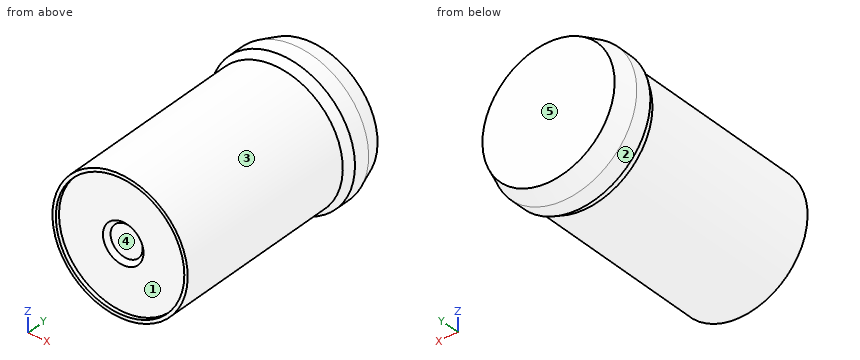
from build123d import *

# Parameters (mm, degrees)
FILLET1_SIZE = 1.5


with BuildPart() as part:
    # Sketch1 → Revolve1 (revolve)
    with BuildSketch(Plane.XY, mode=Mode.PRIVATE) as revolve1_sk:
        Polygon((20, 0), (20, 56.727116956), (21.5, 59.325193167), (21.5, 64.325193167), (19.547262907, 69.998535907), (0, 69.998535907), (0, 2.4), (4.5, 2.4), (4.5, 1.15), (19, 1.15), (19, 0), align=None)
    revolve(revolve1_sk.sketch.rotate(Axis((0, 2.4, 0), (0, 1, 0)), 90), axis=Axis((0, 2.4, 0), (0, 1, 0)))

    # Fillet1
    # the kernel refuses this chamfer: 1.5 mm, written as the material it takes off along each edge
    with BuildSketch(Plane(origin=(0, 1.15, 0), x_dir=(0, 0, -1), z_dir=(1, 0, 0))) as fillet1_piece_1_section:
        Polygon((4.5, FILLET1_SIZE), (4.5 + FILLET1_SIZE, 0), (4.5, 0), align=None)
    fillet1_piece_1 = revolve(axis=Axis((0, 1.15, 0), (0, 1, 0)), mode=Mode.PRIVATE)
    fillet1_piece_1 = split(fillet1_piece_1, bisect_by=Plane(origin=(0, 2.4, 5.37255081), z_dir=(0, -1, 0)), keep=Keep.TOP, mode=Mode.PRIVATE)
    add(fillet1_piece_1, mode=Mode.SUBTRACT)


solid = part.part
The model under review builds one solid part; all positions refer to its coordinate system, in mm. Face numbers are marked on the shaded views. A direction names the side the tool comes from. Give positions to 0.01 mm unless a question says otherwise; leave off trailing zeros. Order: outer loops, then holes, each group sorted by start corner. A loop starts at its lowest first (then second) coordinate and runs counter-clockwise, first axis right, second up. Notation, with made-up numbers: M 75,21.25 L 93,21.25 A28 ccw 93,55.25 Z; hole C 6,5.5 d9. An arc over 180 degrees is marked long. Use one line per item in the form item = value. Start each with the question number.
Item 1: We need section A-A on x = 0. Give the boundary of the cut face in (y, z).
Item 2: Insertion check: pin 1 Ø5 at (x, y) = (15.5, 14) entering from -Z; pin 2 Ø10 at (x, z) = (11, 6.5) entering from -Y; pin 3 Ø1.5 at (y, z) = (10.5, 6) entering from -X. Each pin has a flat end and moves straight along its axis. Give the tip position at first contact, or say it passes through.
Item 3: We need section C-C on y = 21. Give the boundary of the cut face in (x, z).
Item 4: To check wall thickness, follow line 1 along X through (y, z) = (0.95, 0); line 2 along Y through (x, z) = (14, -7); line 3 along X through (y, z) = (41, 10.5). State the ranges of each line that lie inside material, in increasing order. Write a range as from..to.
Item 5: We need section B-B on z = 0. Give the boundary of the cut face in (x, y).
Item 6: The part is to be moulded in two halves that separate along Z. For the marked faces 3, 4 and 5, say which applies: pulls with the +Z half, pulls with the -Z half, needs draft (parallel to the pull), parting line crosses it, or undercut.
Item 7: For the marked faces 1 and 2, list the 3-axis set-ups (+Z, -Z, +X, -X, +Y, -Y) from which the entire face can be reached by the end or side of a thin tool; tool diameter is ignored.
Completed:
q1.outline = M 0,-20 L 56.73,-20 L 59.33,-21.5 L 64.33,-21.5 L 70,-19.55 L 70,19.55 L 64.33,21.5 L 59.33,21.5 L 56.73,20 L 0,20 L 0,19 L 1.15,19 L 1.15,6 L 2.4,4.75 L 2.4,-4.75 L 1.15,-6 L 1.15,-19 L 0,-19 Z
q2.pin_1 = -15.2
q2.pin_2 = 1.15
q2.pin_3 = -19.3
q3.outline = C 0,0 d40
q4.line_1 = -20..-19, 19..20
q4.line_2 = 1.15..70
q4.line_3 = -17.02..17.02
q5.outline = M -21.5,59.33 L -20,56.73 L -20,0 L -19,0 L -19,1.15 L -6,1.15 L -4.75,2.4 L 4.75,2.4 L 6,1.15 L 19,1.15 L 19,0 L 20,0 L 20,56.73 L 21.5,59.33 L 21.5,64.33 L 19.55,70 L -19.55,70 L -21.5,64.33 Z
q6.face_3 = parting line crosses it
q6.face_4 = undercut
q6.face_5 = needs draft
q7.face_1 = -Y
q7.face_2 = +Y, -Y
